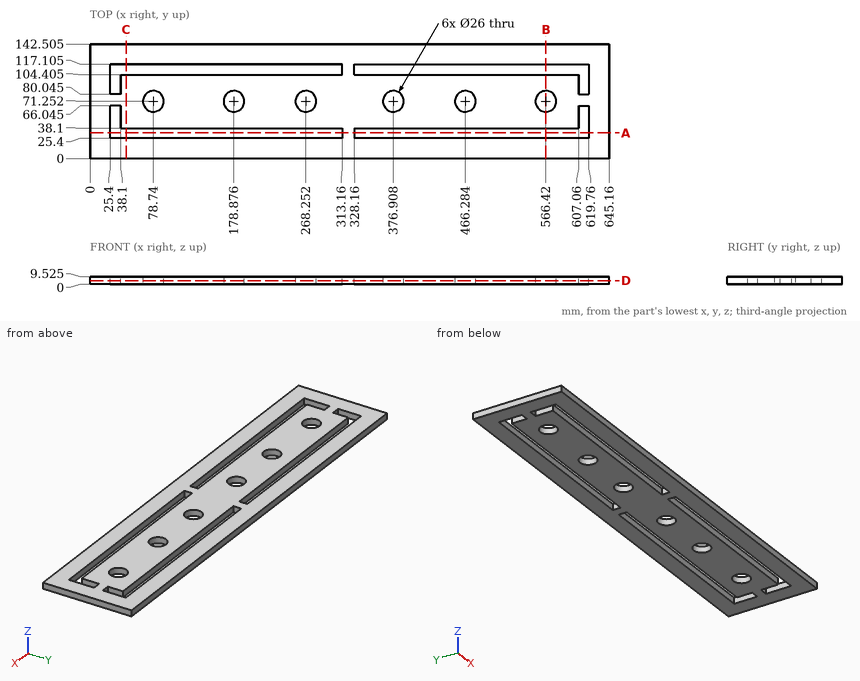
Geometry: see drawing. Coordinates: mm, zero at the bounding-box minimum. Coordinates: 2 decimals unless noted, no trailing zeros. Loops run counter-clockwise (first coordinate to the right, second up) from the corner with the lowest first, then second, coordinate; pieces in that order, holes last. Notation, with made-up numbers: (-31.75, -2.75) -> (3.25, -2.75) arc R17 ccw to (3.25, 21.25) -> close; hole circle Ø11 at (-13, 8). An arc over 180 degrees is marked (long way). Write item = value, one per line. Start each with the question number.
Item 1: Cut plane C-C, the plane x = 45. Return loops of the section in (y, z) (1 decimal).
Item 2: Material intervals for line 1 (Y direction, x = 238, z = 7.25) (1 decimal); line 2 (Y direction, x = 566.42, z = 5.25) (1 decimal); line 3 (Y direction, x = 178, z = 1) (1 decimal), sorted ascending.
Item 3: Cut plane D-D, the plane z = 4.5. Count the separate pieces of the cut face and the enclosed holes in it, plus the area to 3 significant figures.
Item 4: Cut plane A-A, the plane y = 32. Return loops of the section in (x, z) (1 decimal), plus the area to 3 significant figures.
Item 5: Cut plane B-B, the plane x = 566.42. Return loops of the section in (y, z) (1 decimal), plus the area to 3 significant figures.
Item 6: First-contact query: P1, Ø3, axis at y = 111, z = 4.5, coming from the -X side. Flat tip, straight axial feed; report the tip coordinate or a pass-through.
Ans:
q1.outline = (0, 0) -> (25.4, 0) -> (25.4, 9.5) -> (0, 9.5) -> close; (38.1, 0) -> (104.4, 0) -> (104.4, 9.5) -> (38.1, 9.5) -> close; (117.1, 0) -> (142.5, 0) -> (142.5, 9.5) -> (117.1, 9.5) -> close
q2.line_1 = 0 to 25.4, 38.1 to 104.4, 117.1 to 142.5
q2.line_2 = 0 to 25.4, 38.1 to 58.3, 84.3 to 104.4, 117.1 to 142.5
q2.line_3 = 0 to 25.4, 38.1 to 58.3, 84.2 to 104.4, 117.1 to 142.5
q3.separate_pieces = 1
q3.enclosed_holes = 10
q3.area = 72,700 mm²
q4.outline = (0, 0) -> (25.4, 0) -> (25.4, 9.5) -> (0, 9.5) -> close; (313.2, 0) -> (328.2, 0) -> (328.2, 9.5) -> (313.2, 9.5) -> close; (619.8, 0) -> (645.2, 0) -> (645.2, 9.5) -> (619.8, 9.5) -> close
q4.area = 627 mm²
q5.outline = (0, 0) -> (25.4, 0) -> (25.4, 9.5) -> (0, 9.5) -> close; (38.1, 0) -> (58.3, 0) -> (58.3, 9.5) -> (38.1, 9.5) -> close; (84.3, 0) -> (104.4, 0) -> (104.4, 9.5) -> (84.3, 9.5) -> close; (117.1, 0) -> (142.5, 0) -> (142.5, 9.5) -> (117.1, 9.5) -> close
q5.area = 868 mm²
q6.P1 = 0
